from build123d import *

# Parameters (mm, degrees)
SKETCH_1_W          = 350
SKETCH_1_H          = 101.37
EXTRUDE_1_DEPTH     = 3
SKETCH_2_R          = 3
SKETCH_2_W          = 20
SKETCH_2_H          = 20
CUT_EXTRUDE_1_DEPTH = 183.21681927
FILLET_1_R          = 30


with BuildPart() as part:
    # 草圖1 → 填料-伸長1 (new body)
    with BuildSketch(Plane(origin=(0, 0, 0), x_dir=(1, 0, 0), z_dir=(0, 1, 0))):
        Rectangle(SKETCH_1_W, SKETCH_1_H)
    extrude(amount=EXTRUDE_1_DEPTH)

    # 草圖2 → 除料-伸長1 (cut, through all)
    with BuildSketch(Plane(origin=(0, 3, 0), x_dir=(1, 0, 0), z_dir=(0, 1, 0))):
        with Locations(Location((-87.5, 40.685, 0), (0, 0, 270))):
            Circle(SKETCH_2_R)
        with Locations(Location((0, 40.685, 0), (0, 0, 270))):
            Circle(SKETCH_2_R)
        with Locations(Location((87.5, 40.685, 0), (0, 0, 270))):
            Circle(SKETCH_2_R)
        with Locations((-165, 40.685)):
            Rectangle(SKETCH_2_W, SKETCH_2_H)
        with Locations((165, 40.685)):
            Rectangle(SKETCH_2_W, SKETCH_2_H)
    extrude(amount=-CUT_EXTRUDE_1_DEPTH, mode=Mode.SUBTRACT)

    # 圓角1
    fillet_1_edges = [part.edges().sort_by_distance(p)[0] for p in [
        (175, 1.5, 50.685),
        (-175, 1.5, 50.685),
    ]]
    fillet(fillet_1_edges, radius=FILLET_1_R)


solid = part.part
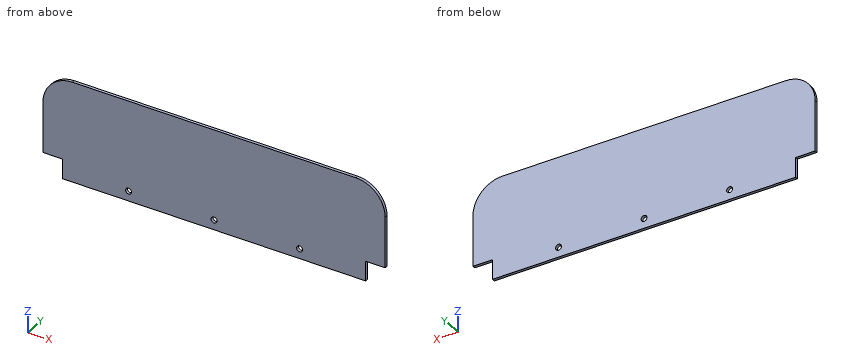
Build history of the part. All positions in model axes, mm. Round coordinates to 2 decimals unless told otherwise and drop trailing zeros. Loops run counter-clockwise (first coordinate to the right, second up) from the corner with the lowest first, then second, coordinate; pieces in that order, holes last. Notation, with made-up numbers: (-2, -17.75) -> (29, -17.75) arc R20 ccw to (29, -8.75) -> close; hole circle Ø10 at (-3.5, 28). An arc over 180 degrees is marked (long way). Answer in a Markdown table with one row per item.
Item 1: Saw through at C-C (z = 39.5). Write the cut outline in (x, y).
Answers below:
| item | result |
|---|---|
| outline | (-168.37, 0) -> (168.37, 0) -> (168.37, 3) -> (-168.37, 3) -> close |
Item 2: Pin check, flat tips, straight feed: pin 1 (5.5 mm diameter, centred on x = 87.5, z = -40.685, fed in from -Y); pin 2 (12 mm diameter, centred on x = 105.5, z = -4.5, fed in from -Y); pin 3 (0.9 mm diameter, centred on x = 160.5, y = 1.5, fed in from -Z) (3 decimals). Stop position of each tip, or through.
Answers below:
| item | result |
|---|---|
| pin 1 | passes through |
| pin 2 | stops at y = 0 |
| pin 3 | stops at z = -30.685 |
Item 3: Saw through at A-A (y = 1.5). Write the cut outline in (x, z) (3 decimals), and give its area (3 significant figures).
Answers below:
| item | result |
|---|---|
| outline | (-175, -30.685) -> (-155, -30.685) -> (-155, -50.685) -> (155, -50.685) -> (155, -30.685) -> (175, -30.685) -> (175, 20.685) arc R30 ccw to (145, 50.685) -> (-145, 50.685) arc R30 ccw to (-175, 20.685) -> close; hole circle Ø6 at (-87.5, -40.685); hole circle Ø6 at (0, -40.685); hole circle Ø6 at (87.5, -40.685) |
| area | 34,200 mm² |
Item 4: Drill centre lines: L1, parallel to X at y = 1.1, z = -38; L2, parallel to X at y = 1.5, z = -34; L3, parallel to X at y = 1.7, z = 34.5. Where is each one in solid material? Low to high. Write a range as [from, to].
Answers below:
| item | result |
|---|---|
| L1 | x = [-155, -88.84], [-86.16, -1.34], [1.34, 86.16], [88.84, 155] |
| L2 | x = [-155, 155] |
| L3 | x = [-171.63, 171.63] |
Item 5: Saw through at B-B (x = 0). Write the cut outline in (y, z) (3 decimals), and give its area (3 significant figures).
Answers below:
| item | result |
|---|---|
| outline | (0, -50.685) -> (3, -50.685) -> (3, -43.685) -> (0, -43.685) -> close; (0, -37.685) -> (3, -37.685) -> (3, 50.685) -> (0, 50.685) -> close |
| area | 286 mm² |
